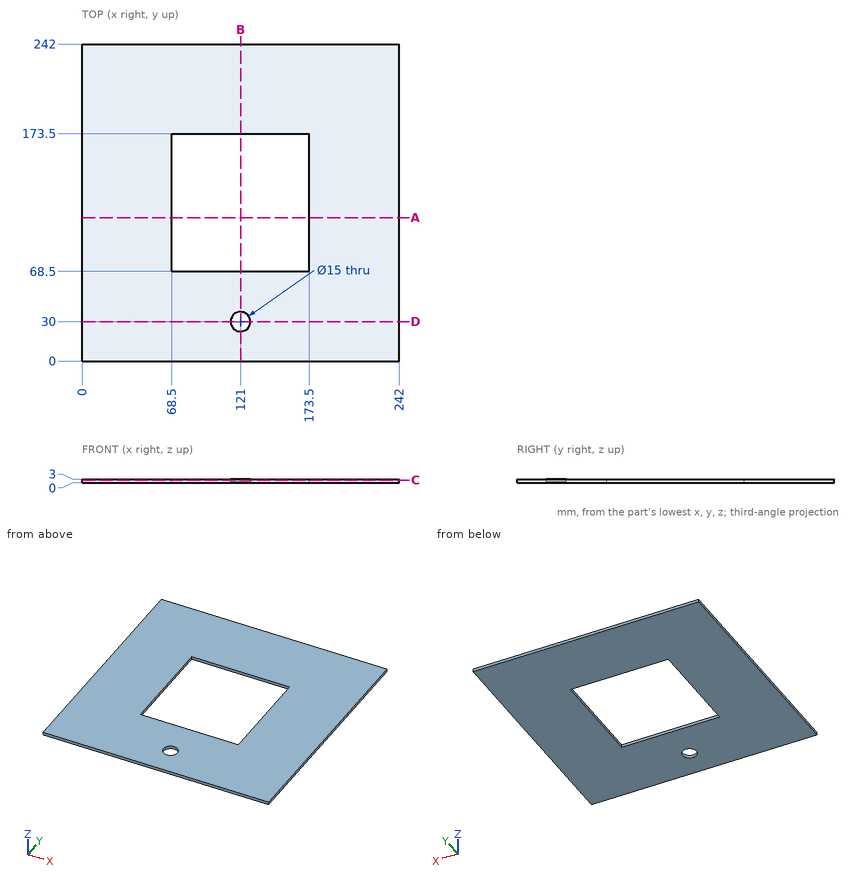
The figure shows three views and two pictorial views of one solid part (mm, origin at its lowest corner). Answer the questions. Give positions to 0.01 mm unless a question says otherwise; leave off trailing zeros. Order: outer loops, then holes, each group sorted by start corner. A loop starts at its lowest first (then second) coordinate and runs counter-clockwise, first axis right, second up. Notation, with made-up numbers: M 0.25,-33 L 49.25,-33 A22 ccw 49.25,-21 Z; hole C 70.25,9.25 d6. An arc over 180 degrees is marked long. Return JSON: item names as keys, results as strings.
1) Straight lines are drawn through the part: line 1 along Y through (x, z) = (121, 2.4); line 2 along Y through (x, z) = (78.5, 2.15). For each, find the intervals that lie inside material, in ascending order. Write a range as [from, to].
Resolved:
{"line 1": "[0, 22.5], [37.5, 68.5], [173.5, 242]", "line 2": "[0, 68.5], [173.5, 242]"}
2) Section D-D, the plane y = 30 is taken. Write down the section's boundary in (x, z).
Resolved:
{"outline": "M 0,0 L 113.5,0 L 113.5,3 L 0,3 Z; M 128.5,0 L 242,0 L 242,3 L 128.5,3 Z"}
3) Section C-C, the plane z = 2.1 is taken. Write down the section's boundary in (x, y).
Resolved:
{"outline": "M 0,0 L 242,0 L 242,242 L 0,242 Z; hole M 68.5,68.5 L 173.5,68.5 L 173.5,173.5 L 68.5,173.5 Z; hole C 121,30 d15"}
4) Section A-A, the plane y = 109.5 is taken. Write down the section's boundary in (x, z).
Resolved:
{"outline": "M 0,0 L 68.5,0 L 68.5,3 L 0,3 Z; M 173.5,0 L 242,0 L 242,3 L 173.5,3 Z"}
5) Section B-B, the plane x = 121 is taken. Write down the section's boundary in (y, z).
Resolved:
{"outline": "M 0,0 L 22.5,0 L 22.5,3 L 0,3 Z; M 37.5,0 L 68.5,0 L 68.5,3 L 37.5,3 Z; M 173.5,0 L 242,0 L 242,3 L 173.5,3 Z"}
